The listing builds one solid part. Answer for the finished solid, in the listing's coordinates (mm). Face numbers are marked on the shaded views. Coordinates: 2 decimals unless noted, no trailing zeros. Loops run counter-clockwise (first coordinate to the right, second up) from the corner with the lowest first, then second, coordinate; pieces in that order, holes last. Notation, with made-up numbers: (-7.5, 75) - (17.5, 75) arc R21 ccw to (17.5, 103) - close; hole circle Ø2 at (84, 79). An arc over 180 degrees is marked (long way). Return JSON: item names as keys, results as strings. Group by question number.
1. Find the intervals of material crossed by line 1 along Z through (x, y) = (0, 3.4); line 2 along Z through (x, y) = (0, 0.25); line 3 along Y through (x, z) = (-6.75, -4), in increasing order.
2. Section B-B (x = 0) is taken. Write down the section's boundary in (y, z).
3. The mould has two halves that part along Z. Classify the marked faces 1, 2 and 3: pulls with the +Z half, pulls with the -Z half, needs draft (parallel to the pull), parting line crosses it, or undercut.
4. Section D-D (z = 8.25) is taken. Write down the section's boundary in (x, y).
5. Section A-A (z = 0) is taken. Write down the section's boundary in (x, y), and give its area (3 significant figures).
6. Section C-C (y = -2) is taken. Write down the section's boundary in (x, z).
7. Each of these flat-tipped pins is pushed along its axis until it touches: P1, Ø2, axis at x = 6.5, y = 1, coming from the -Z side; P2, Ø1.5, axis at y = 1, z = -6, coming from the -X side; P3, Ø2, axis at x = 1.5, z = -0.5, coming from the +Y side. Where does it stop, or does it pass through?
```python
from build123d import *

# Parameters (mm, degrees)
F0_R     = 5
F0_R_2   = 4
F1_DEPTH = 3.5
F0_R_3   = 11
F0_R_4   = 10
F2_DEPTH = 3.25


with BuildPart() as f1:
    # F0 (on Front) → F1 (new body, symmetric)
    with BuildSketch(Plane.XZ):
        Circle(F0_R)
        Circle(F0_R_2, mode=Mode.SUBTRACT)
    extrude(amount=F1_DEPTH, both=True)



with BuildPart() as f1b:
    # F0 (on Front) → F1, piece 2 (new body, symmetric)
    with BuildSketch(Plane.XZ):
        Circle(F0_R_3)
        Circle(F0_R_4, mode=Mode.SUBTRACT)
    extrude(amount=F1_DEPTH, both=True)


with BuildPart() as f1_1:
    add(f1.part)

    add(f1b.part)  # F2 merges F1b
    # F0 (on Front) → F2 (join, symmetric)
    with BuildSketch(Plane.XZ):
        Circle(F0_R_4)
        Circle(F0_R, mode=Mode.SUBTRACT)
    extrude(amount=F2_DEPTH, both=True)


solid = f1_1.part
```
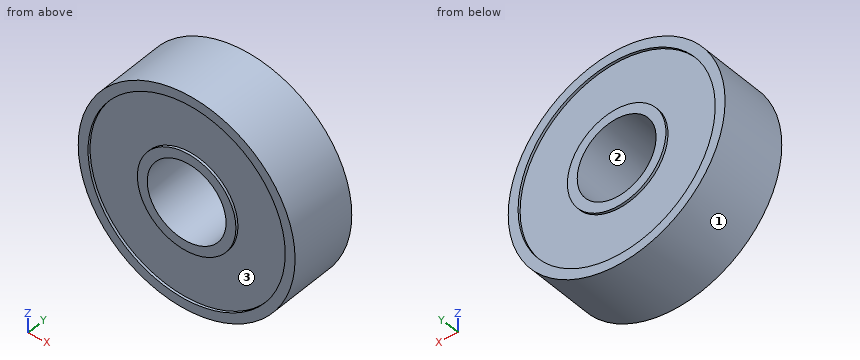
The answers:
{
 "1": {"line 1": "z = -11 to -10, -5 to -4, 4 to 5, 10 to 11", "line 2": "z = -11 to -4, 4 to 11", "line 3": "y = -3.25 to 3.25"},
 "2": {"outline": "(-3.5, -11) - (3.5, -11) - (3.5, -10) - (3.25, -10) - (3.25, -5) - (3.5, -5) - (3.5, -4) - (-3.5, -4) - (-3.5, -5) - (-3.25, -5) - (-3.25, -10) - (-3.5, -10) - close; (-3.5, 4) - (3.5, 4) - (3.5, 5) - (3.25, 5) - (3.25, 10) - (3.5, 10) - (3.5, 11) - (-3.5, 11) - (-3.5, 10) - (-3.25, 10) - (-3.25, 5) - (-3.5, 5) - close"},
 "3": {"face 1": "parting line crosses it", "face 2": "undercut", "face 3": "undercut"},
 "4": {"outline": "(-7.28, -3.5) - (-5.65, -3.5) - (-5.65, -3.25) - (5.65, -3.25) - (5.65, -3.5) - (7.28, -3.5) - (7.28, 3.5) - (5.65, 3.5) - (5.65, 3.25) - (-5.65, 3.25) - (-5.65, 3.5) - (-7.28, 3.5) - close"},
 "5": {"outline": "(-11, -3.5) - (-10, -3.5) - (-10, -3.25) - (-5, -3.25) - (-5, -3.5) - (-4, -3.5) - (-4, 3.5) - (-5, 3.5) - (-5, 3.25) - (-10, 3.25) - (-10, 3.5) - (-11, 3.5) - close; (4, -3.5) - (5, -3.5) - (5, -3.25) - (10, -3.25) - (10, -3.5) - (11, -3.5) - (11, 3.5) - (10, 3.5) - (10, 3.25) - (5, 3.25) - (5, 3.5) - (4, 3.5) - close", "area": "93.0 mm2"},
 "6": {"outline": "circle Ø22 at (0, 0); hole circle Ø8 at (0, 0)"},
 "7": {"P1": "stops at z = -9.53", "P2": "stops at x = -9.67", "P3": "passes through"}
}
